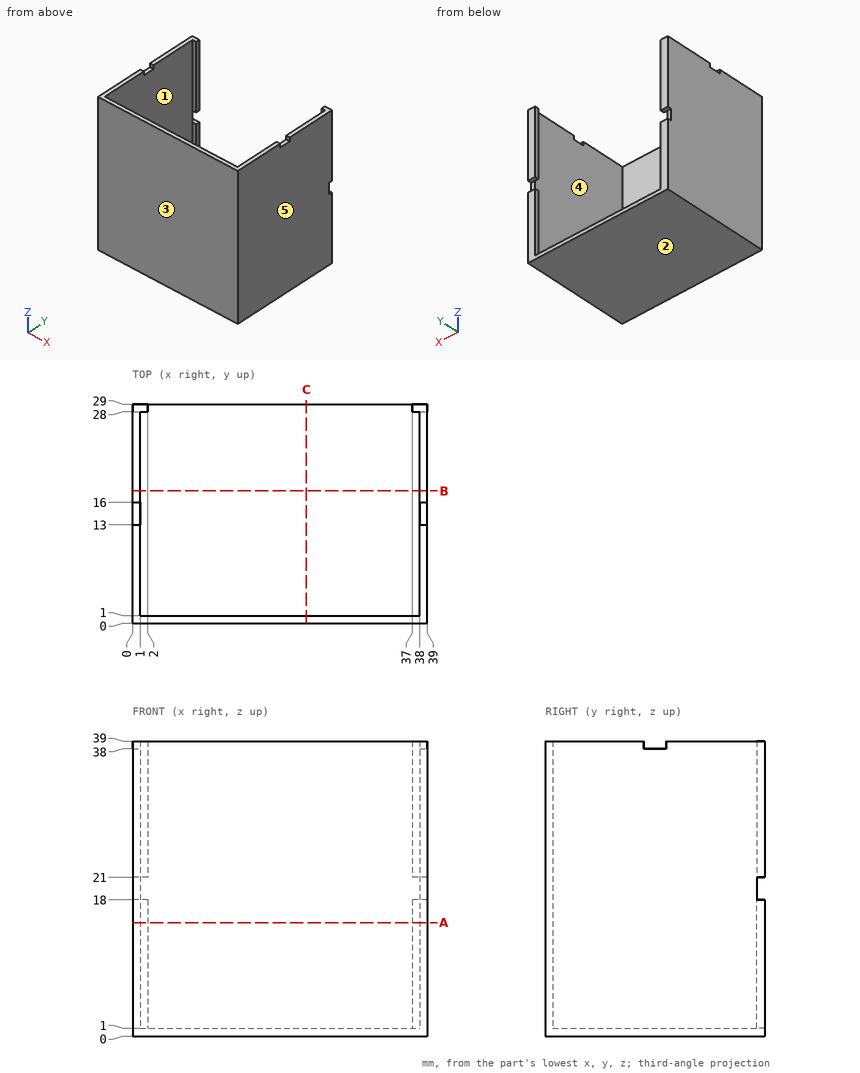
Here's the drawing with two shaded views (mm, measured from the low corner). I have some questions. A direction names the side the tool comes from. Give positions to 0.01 mm unless a question says otherwise; leave off trailing zeros. Write each loop counter-clockwise with the first axis right and the second up, starting at its lowest first coordinate (ties: lowest second). Pieces come first, ordered by that corner, then holes. Notation, with made-up numbers: (67.5, 21.25) -> (97.5, 21.25) arc R15 cw to (97.5, 37.25) -> close; hole circle Ø7 at (84, 78.5). An arc over 180 degrees is marked (long way). Use one line per item in the form item = value.
1) Suppose I cut it at B-B (y = 17.5). Please give me the cut outline in (x, z).
Verdict:
outline = (0, 0) -> (39, 0) -> (39, 39) -> (38, 39) -> (38, 1) -> (1, 1) -> (1, 39) -> (0, 39) -> close
2) If I drill on L1, parallel to X at y = 4.5, z = 36; L2, parallel to Z at x = 25.5, y = 27.75, over which ranges is the centre line in solid material (lowest first)? Write a range as [from, to].
Verdict:
L1 = [0, 1], [38, 39]
L2 = [0, 1]
3) We'd pull the mould along Y, two halves only. Please class the marked faces 3, 4 and 5: +Y half, -Y half, draft (parallel to the pull), parting line (faces both ways), or undercut.
Verdict:
face_3 = -Y half
face_4 = undercut
face_5 = draft
4) Suppose I cut it at C-C (x = 23). Please give me the cut outline in (y, z).
Verdict:
outline = (0, 0) -> (29, 0) -> (29, 1) -> (1, 1) -> (1, 39) -> (0, 39) -> close
5) I'm going to push flat-ended pins straight in: pin 1 (8 mm diameter, centred on x = 20.5, z = 32, fed in from +Y); pin 2 (0.5 mm diameter, centred on x = 38.5, y = 14, fed in from +Z); pin 3 (1.1 mm diameter, centred on x = 38.5, z = 19, fed in from +Y). Where does each tip first touch, or does it pass through?
Verdict:
pin_1 = 1
pin_2 = 38
pin_3 = 28
6) Suppose I cut it at A-A (z = 15). Please give me the cut outline in (x, y).
Verdict:
outline = (0, 0) -> (39, 0) -> (39, 29) -> (37, 29) -> (37, 28) -> (38, 28) -> (38, 1) -> (1, 1) -> (1, 28) -> (2, 28) -> (2, 29) -> (0, 29) -> close
7) On a 3-axis mill with a long thin cutter (end or side, diameter ignored), from which of +Z, -Z, +X, -X, +Y, -Y can I reach the whole of each face in a straight line? I mean the marked faces 1 and 2. Say none if no direction works.
Verdict:
face_1 = +Z
face_2 = -Z, +X, -X, +Y, -Y
